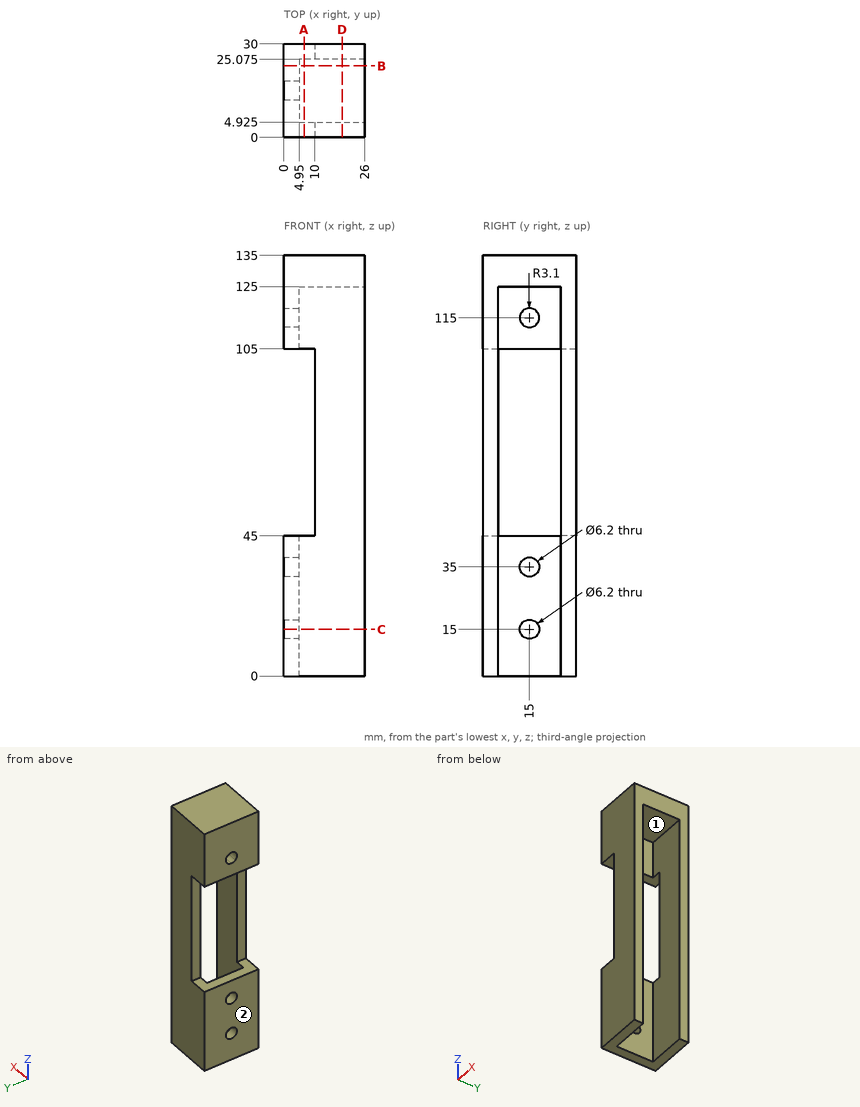
Geometry: see drawing. Coordinates: mm, zero at the bounding-box minimum. A direction names the side the tool comes from. Give positions to 0.01 mm unless a question says otherwise; leave off trailing zeros. Loops run counter-clockwise (first coordinate to the right, second up) from the corner with the lowest first, then second, coordinate; pieces in that order, holes last. Notation, with made-up numbers: M 55.5,44 L 96.5,44 A26 cw 96.5,61 Z; hole C -10,-7.75 d11. An arc over 180 degrees is marked long. Answer as CSV lines item,"result". Start each with the question number.
1. Reachability of the marked faces 1 and 2 from +Z, -Z, +X, -X, +Y, -Y: full face, straight path, thin tool, end or side. Return the list, or none.
2. Section D-D on x = 18.75. Return loops of the section in (y, z) (3 decimals).
3. Section C-C on z = 15. Return loops of the section in (x, y) (3 decimals), plus the area to 3 significant figures.
4. Section A-A on x = 6.5. Return loops of the section in (y, z) (3 decimals), plus the area to 3 significant figures.
5. Section B-B on y = 23. Return loops of the section in (x, z).
6. Line query: L1, parallel to Y at x = 2.9, z = 35; L2, parallel to Y at x = 24.75, z = 110 (3 decimals); L3, parallel to X at y = 4.75, z = 64. Output: solid intervals per line, ascending.
7. Pin query (flat end, axial travel): P1, Ø2.5, axis at y = 27, z = 68.5, coming from the -X side; P2, Ø5, axis at y = 15, z = 35, coming from the +X side; P3, Ø5, axis at x = 9, z = 49, coming from the -Y side; P4, Ø16, axis at y = 16, z = 116.5, coming from the +X side. Return the tip coordinate at first contact, or that it passes through.
Computed values:
1,face 1,"-Z, +X"
1,face 2,"+Z, -Z, -X, +Y, -Y"
2,outline,"M 0,0 L 4.925,0 L 4.925,125 L 25.075,125 L 25.075,0 L 30,0 L 30,135 L 0,135 Z"
3,outline,"M 0,0 L 26,0 L 26,4.925 L 4.95,4.925 L 4.95,11.9 L 0,11.9 Z; M 0,18.1 L 4.95,18.1 L 4.95,25.075 L 26,25.075 L 26,30 L 0,30 Z"
3,area,"325 mm²"
4,outline,"M 0,0 L 4.925,0 L 4.925,45 L 0,45 Z; M 0,105 L 4.925,105 L 4.925,125 L 25.075,125 L 25.075,105 L 30,105 L 30,135 L 0,135 Z; M 25.075,0 L 30,0 L 30,45 L 25.075,45 Z"
4,area,"940 mm²"
5,outline,"M 0,0 L 4.95,0 L 4.95,45 L 0,45 Z; M 0,105 L 4.95,105 L 4.95,125 L 26,125 L 26,135 L 0,135 Z"
6,L1,"y = 0 to 11.9, 18.1 to 30"
6,L2,"y = 0 to 4.925, 25.075 to 30"
6,L3,"x = 10 to 26"
7,P1,"stops at x = 10"
7,P2,"passes through"
7,P3,"stops at y = 0"
7,P4,"stops at x = 4.95"
